The listing builds one solid part. Answer for the finished solid, in the listing's coordinates (mm). Face numbers are marked on the shaded views. Give positions to 0.01 mm unless a question says otherwise; leave off trailing zeros. Loops run counter-clockwise (first coordinate to the right, second up) from the corner with the lowest first, then second, coordinate; pieces in that order, holes last. Notation, with made-up numbers: (75, 53.5) - (125, 53.5) arc R17 cw to (125, 71.5) - close; hole circle Ø6 at (-22, -1). An arc over 180 degrees is marked (long way). Write item = value, one per line. Start each with the question number.
1) The part is cut by section C-C on y = 9. Write down the section's boundary in (x, z), plus the area to 3 significant figures.
2) Flat-ended cylindrical pins translate along their axes: P1, Ø2, axis at x = -16, z = 32, coming from the -Y side; P2, Ø6, axis at x = 43.5, z = 30.5, coming from the -Y side; P3, Ø3, axis at x = -4.5, z = -43.5, coming from the +Y side. Find the tip coordinate at first contact, or state that the pin passes through.
3) Consider probe 1 along X at (y, z) = (10.75, -3); probe 2 along Z at (x, y) = (0, 6.2); probe 3 along Y at (x, z) = (3, 11). Determine where each line is inside the solid, lowest interval first.
4) The mould has two halves that part along Z. Classify the marked faces 1, 2, 3 and 4: +Z half, -Z half, draft (parallel to the pull), parting line (faces both ways), or undercut.
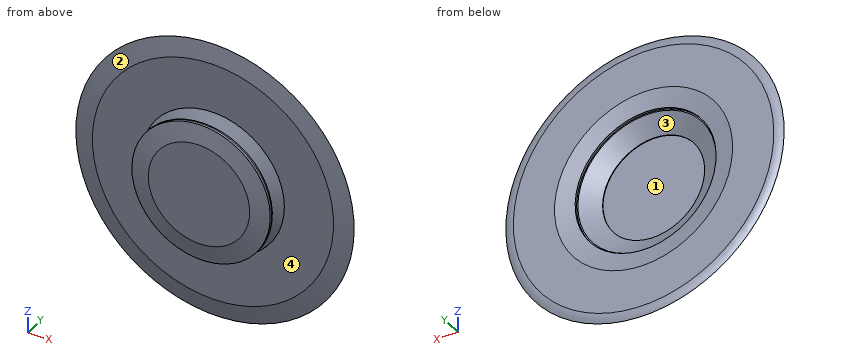
from build123d import *

# Parameters (mm, degrees)
SKETCH1_R           = 41.369507048
BOSS_EXTRUDE1_DEPTH = 15
SKETCH3_R           = 27.5
CUT_EXTRUDE1_DEPTH  = 9
SKETCH4_R           = 41.369507048
CUT_EXTRUDE2_DEPTH  = 5
SKETCH5_R           = 53.188342474
BOSS_EXTRUDE2_DEPTH = 2
SKETCH6_R           = 40
CUT_EXTRUDE8_DEPTH  = 2
FILLET1_R           = 10
FILLET3_R           = 5
SKETCH7_R           = 75
BOSS_EXTRUDE3_DEPTH = 3
SKETCH8_R           = 38
CUT_EXTRUDE11_DEPTH = 3
CHAMFER4_SIZE       = 10
CHAMFER4_SIZE2      = 1.763269807
CHAMFER5_SIZE       = 10
CHAMFER5_SIZE2      = 1.763269807
FILLET5_R           = 10
SKETCH10_R          = 37.303847577
BOSS_EXTRUDE4_DEPTH = 5
CHAMFER6_SIZE       = 10
CHAMFER6_SIZE2      = 1.763269807
FILLET6_R           = 2


with BuildPart() as part:
    # Sketch1 → Boss-Extrude1 (new body)
    with BuildSketch(Plane(origin=(0, 0, 0), x_dir=(1, 0, 0), z_dir=(0, 1, 0))):
        with Locations(Location((0, 0, 0), (0, 0, 270))):
            Circle(SKETCH1_R)
    extrude(amount=BOSS_EXTRUDE1_DEPTH)

    # Sketch3 → Cut-Extrude1 (cut)
    with BuildSketch(Plane(origin=(0, 15, 0), x_dir=(1, 0, 0), z_dir=(0, 1, 0))):
        with Locations(Location((0, 0, 0), (0, 0, 270))):
            Circle(SKETCH3_R)
    extrude(amount=-CUT_EXTRUDE1_DEPTH, mode=Mode.SUBTRACT)

    # Sketch4 → Cut-Extrude2 (cut)
    with BuildSketch(Plane(origin=(0, 0, 0), x_dir=(1, 0, 0), z_dir=(0, 1, 0))):
        with Locations(Location((0, 0, 0), (0, 0, 270))):
            Circle(SKETCH4_R)
    extrude(amount=CUT_EXTRUDE2_DEPTH, mode=Mode.SUBTRACT)

    # Chamfer2: read off the stored shape, not the designer's step
    # Chamfer2 outline → Chamfer2 (revolve, cut)
    with BuildSketch(Plane.XY):
        Polygon((26.369507048, 5), (41.369507048, 5), (41.369507048, 13.660254038), align=None)
        Polygon((27.5, 6.339745962), (41.369507048, 14.34730959), (41.369507048, 15), (27.5, 15), align=None)
    revolve(axis=Axis((0, 0, 0), (0, 1, 0)), mode=Mode.SUBTRACT)

    # Sketch5 → Boss-Extrude2 (add)
    with BuildSketch(Plane(origin=(0, 15, 0), x_dir=(1, 0, 0), z_dir=(0, 1, 0))):
        with Locations(Location((0, 0, 0), (0, 0, 270))):
            Circle(SKETCH5_R)
    extrude(amount=-BOSS_EXTRUDE2_DEPTH)

    # Sketch6 → Cut-Extrude8 (cut)
    with BuildSketch(Plane(origin=(0, 15, 0), x_dir=(1, 0, 0), z_dir=(0, 1, 0))):
        with Locations(Location((0, 0, 0), (0, 0, 270))):
            Circle(SKETCH6_R)
    extrude(amount=-CUT_EXTRUDE8_DEPTH, mode=Mode.SUBTRACT)

    # Fillet1
    # the kernel refuses this fillet: 10 mm, written as the material it takes off along each edge
    with BuildSketch(Plane(origin=(0, 15, 0), x_dir=(0, 0, 1), z_dir=(-1, 0, 0))) as fillet1_piece_1:
        with BuildLine():
            CenterArc((46, -10), FILLET1_R, 90, 36.869897646)
            Line((40, -2), (39.88, -1.84))
            ThreePointArc((39.88, -1.84), (39.8, -1), (39.8, 0))
            Line((39.8, 0), (40, 0.2))
            Line((40, 0.2), (46, 0.2))
            Line((46, 0.2), (46, 0))
        make_face()
    revolve(axis=Axis((0, 15, 0), (0, 1, 0)), mode=Mode.SUBTRACT)

    # Fillet3
    # the kernel refuses this fillet: 5 mm, written as the material it takes off along each edge
    with BuildSketch(Plane(origin=(0, 15, 0), x_dir=(0, 0, 1), z_dir=(-1, 0, 0))) as fillet3_piece_1:
        with BuildLine():
            CenterArc((49.188342474, -5), FILLET3_R, 36.869897646, 53.130102354)
            Line((49.188342474, 0), (49.188342474, 0.1))
            Line((49.188342474, 0.1), (53.188342474, 0.1))
            Line((53.188342474, 0.1), (53.288342474, 0))
            ThreePointArc((53.288342474, 0), (53.288342474, -1), (53.268342474, -1.94))
            Line((53.268342474, -1.94), (53.188342474, -2))
        make_face()
    revolve(axis=Axis((0, 15, 0), (0, 1, 0)), mode=Mode.SUBTRACT)

    # Sketch7 → Boss-Extrude3 (add)
    with BuildSketch(Plane(origin=(0, 15, 0), x_dir=(1, 0, 0), z_dir=(0, 1, 0))):
        with Locations(Location((0, 0, 0), (0, 0, 270))):
            Circle(SKETCH7_R)
    extrude(amount=-BOSS_EXTRUDE3_DEPTH)

    # Sketch8 → Cut-Extrude11 (cut)
    with BuildSketch(Plane(origin=(0, 15, 0), x_dir=(1, 0, 0), z_dir=(0, 1, 0))):
        with Locations(Location((0, 0, 0), (0, 0, 270))):
            Circle(SKETCH8_R)
    extrude(amount=-CUT_EXTRUDE11_DEPTH, mode=Mode.SUBTRACT)

    # Chamfer4
    chamfer4_edges = [part.edges().sort_by_distance(p)[0] for p in [
        (0, 15, -38),
    ]]
    chamfer4_side = [part.faces().sort_by_distance(p)[0] for p in [
        (0, 15, -72.878679656),
    ]]
    chamfer(chamfer4_edges, length=CHAMFER4_SIZE, length2=CHAMFER4_SIZE2, reference=chamfer4_side[0])

    # Chamfer5
    chamfer5_edges = [part.edges().sort_by_distance(p)[0] for p in [
        (0, 12, -75),
    ]]
    chamfer5_side = [part.faces().sort_by_distance(p)[0] for p in [
        (0, 12, -72.878679656),
    ]]
    chamfer(chamfer5_edges, length=CHAMFER5_SIZE, length2=CHAMFER5_SIZE2, reference=chamfer5_side[0])

    # Fillet5
    # the kernel refuses this fillet: 10 mm, written as the material it takes off along each edge
    with BuildSketch(Plane(origin=(0, 15, 0), x_dir=(0, 0, 1), z_dir=(-1, 0, 0))) as fillet5_piece_1:
        with BuildLine():
            CenterArc((70.182832545, -10), FILLET5_R, 61.202414485, 28.797585515)
            Line((70.182832545, 0), (70.182832545, 0.2))
            Line((70.182832545, 0.2), (75, 0.2))
            Line((75, 0.2), (75.2, 0))
            ThreePointArc((75.2, 0), (75.2, -0.618365096), (75.096343349, -1.061464797))
            Line((75.096343349, -1.061464797), (75, -1.236730193))
        make_face()
    revolve(axis=Axis((0, 15, 0), (0, 1, 0)), mode=Mode.SUBTRACT)

    # Sketch10 → Boss-Extrude4 (add)
    with BuildSketch(Plane(origin=(0, 0, 0), x_dir=(1, 0, 0), z_dir=(0, 1, 0))):
        with Locations(Location((0, 0, 0), (0, 0, 270))):
            Circle(SKETCH10_R)
    extrude(amount=BOSS_EXTRUDE4_DEPTH)

    # Chamfer6
    chamfer6_edges = [part.edges().sort_by_distance(p)[0] for p in [
        (0, 0, -37.303847577),
    ]]
    chamfer6_side = [part.faces().sort_by_distance(p)[0] for p in [
        (0, 0, 0),
    ]]
    chamfer(chamfer6_edges, length=CHAMFER6_SIZE, length2=CHAMFER6_SIZE2, reference=chamfer6_side[0])

    # Fillet6
    fillet6_edges = [part.edges().sort_by_distance(p)[0] for p in [
        (0, 5, -37.303847577),
    ]]
    fillet(fillet6_edges, radius=FILLET6_R)


solid = part.part
Answer below:
q1.outline = circle Ø66.6 at (0, 0); hole circle Ø64.22 at (0, 0)
q1.area = 245 mm2
q2.P1 = 1.32
q2.P2 = 12
q2.P3 = 14.51
q3.probe_1 = -36.2 to -35.01, 35.01 to 36.2
q3.probe_2 = -28.45 to -27.5, 27.5 to 28.45
q3.probe_3 = 0 to 6
q4.face_1 = undercut
q4.face_2 = parting line
q4.face_3 = undercut
q4.face_4 = draft
